Autodesk Inventor part; units mm, degrees
ref_plane "YZ Plane" through (0, 0, 0) normal (1, 0, 0) x (0, 1, 0)
ref_plane "XZ Plane" through (0, 0, 0) normal (0, 1, 0) x (-1, 0, 0)
ref_plane "XY Plane" through (0, 0, 0) normal (0, 0, 1) x (1, 0, 0)
sketch "Szkic1" plane through (0, 0, 0) normal (0, 1, 0) x (-1, 0, 0)
  arc A0 (10.0623, 3) -> (10.0623, -3) centre (0, 0) ccw
  line L0 (13.3003, 3) -> (13.3003, -3)
  line L1 (13.3003, -3) -> (10.0623, -3)
  line L2 (13.3003, 3) -> (10.0623, 3)
  point P0 (13.3003, 0)
  dimension "d0" = 21
  dimension "d1" = 6
  dimension "d2" = 3.238
extrude "Wyciągnięcie proste1" add sketch "Szkic1" against normal blind 13
sketch "Szkic3" plane through (0, -13, 0) normal (0, -1, 0) x (1, 0, 0)
  circle A0 centre (0, 0) radius 10.5
extrude "Wyciągnięcie proste3" add sketch "Szkic3" along normal blind 104
sketch "Szkic4" plane through (0, -117, 0) normal (0, -1, 0) x (1, 0, 0)
  circle A0 centre (0, 0) radius 12.5
  dimension "d9" = 25
extrude "Wyciągnięcie proste4" add sketch "Szkic4" along normal blind 13
properties part number "wal_czlon_2"
Read the model definition and answer for the solid it produces. Units are mm, in the model's axes. A direction names the side the tool comes from. Round coordinates to 2 decimals unless told otherwise and drop trailing zeros. Write each loop counter-clockwise with the first axis right and the second up, starting at its lowest first coordinate (ties: lowest second). Pieces come first, ordered by that corner, then holes.
Q1. Find section B-B on z = 5.5. Determine the outline of the cut face in (x, y), and give its area (3 significant figures).
Values:
outline: (-11.22, -130) - (11.22, -130) - (11.22, -117) - (8.94, -117) - (8.94, 0) - (-8.94, 0) - (-8.94, -117) - (-11.22, -117) - close
area: 2,380 mm2
Q2. Find section A-A on x = 0. Determine the outline of the cut face in (y, z), and give its area (3 significant figures).
Values:
outline: (-130, -12.5) - (-117, -12.5) - (-117, -10.5) - (0, -10.5) - (0, 10.5) - (-117, 10.5) - (-117, 12.5) - (-130, 12.5) - close
area: 2,780 mm2
Q3. The mould has two halves that part along Y. Classify faces 1 (the face through (0, -130, 0)), 2 (the face through (-13.3, -6, 0)), 3 (the face through (-1, 0, 0)), 4 (the face through (-12, -13, 0)): released by +Y, released by -Y, zero draft, split by the parting line, or undercut.
Values:
face 1: released by -Y
face 2: zero draft
face 3: released by +Y
face 4: undercut
Q4. Flat-ended cylindrical pins translate along their axes: P1, Ø7.5, axis at x = 3.5, z = -4, coming from the +Y side; P2, Ø5, axis at y = -57.5, z = 1, coming from the -X side; P3, Ø3, axis at x = -6, y = -102.5, coming from the -Z side; P4, Ø10, axis at x = -6, y = -49, coming from the +Z side. Find the tip coordinate at first contact, or state that the pin passes through.
Values:
P1: stops at y = 0
P2: stops at x = -10.5
P3: stops at z = -9.49
P4: stops at z = 10.45
Q5. Straight lines are drawn through the part: line 1 (X direction, y = -60, z = -0.25); line 2 (Z direction, x = 7.5, y = -69.5); line 3 (X direction, y = -115.5, z = -1.5). For each, find the intervals that lie inside material, in ascending order.
Values:
line 1: x = -10.5 to 10.5
line 2: z = -7.35 to 7.35
line 3: x = -10.39 to 10.39
Q6. A tool of negligible diameter and unlimited length cuts with its end or side. For faces 5 (the face through (-12, -6, -3)), 6 (the face through (-12, -6, 3)), from which of +Z, -Z, +X, -X, +Y, -Y can it reach the whole face along a straight path? Write none if from no direction.
Values:
face 5: -Z, -X, +Y
face 6: +Z, -X, +Y
Q7. Find section C-C on y = -75.5. Determine the outline of the cut face in (x, z), and give its area (3 significant figures).
Values:
outline: circle Ø21 at (0, 0)
area: 346 mm2
